from build123d import *

# Parameters (mm, degrees)
BOSS_EXTRUDE1_DEPTH = 4
SKETCH2_R           = 1.95
CUT_EXTRUDE1_DEPTH  = 3
FILLET1_R           = 0.25


with BuildPart() as part:
    # Sketch1 → Boss-Extrude1 (new body)
    with BuildSketch(Plane(origin=(0, 0, 0), x_dir=(1, 0, 0), z_dir=(0, 1, 0))):
        Polygon((2.362917062, -1.848410928), (2.782229351, 1.122140739), (0.419312289, 2.970551667), (-2.362917062, 1.848410928), (-2.782229351, -1.122140739), (-0.419312289, -2.970551667), align=None)
    extrude(amount=BOSS_EXTRUDE1_DEPTH)

    # Sketch2 → Cut-Extrude1 (cut)
    with BuildSketch(Plane(origin=(0, 4, 0), x_dir=(1, 0, 0), z_dir=(0, 1, 0))):
        Circle(SKETCH2_R)
    extrude(amount=-CUT_EXTRUDE1_DEPTH, mode=Mode.SUBTRACT)

    # Fillet1
    fillet1_edges = [part.edges().sort_by_distance(p)[0] for p in [
        (-1.95, 4, 0),
    ]]
    fillet(fillet1_edges, radius=FILLET1_R)


solid = part.part
Source: CAD feature listing. Evaluate the final solid. Frame: model axes, mm. A direction names the side the tool comes from. Give positions to 0.01 mm unless a question says otherwise; leave off trailing zeros. Order: outer loops, then holes, each group sorted by start corner. A loop starts at its lowest first (then second) coordinate and runs counter-clockwise, first axis right, second up. Notation, with made-up numbers: (-29, -16.5) -> (-6, -16.5) arc R29 cw to (-6, 16.5) -> close; hole circle Ø8 at (22.5, 38.5). An arc over 180 degrees is marked (long way). Write item = value, one per line.
Item 1: Set-up query: faces 4 (the face through (-1.62, 1.97, 2.03)), 5 (the face through (-1.437, 2.394, -1.318)). Return all of +Z, -Z, +X, -X, +Y, -Y with unobstructed straight access to the full face (end or side cutting, diameter ignored); none if empty.
Check result:
face_4 = +Z, -X, +Y, -Y
face_5 = +Y
Item 2: Section query C-C (z = 0). Output: boundary loops of the cut face in (x, y), then the cut area to 3 significant figures.
Check result:
outline = (-2.62, 0) -> (2.62, 0) -> (2.62, 4) -> (2.2, 4) arc R0.25 ccw to (1.95, 3.75) -> (1.95, 1) -> (-1.95, 1) -> (-1.95, 3.75) arc R0.25 ccw to (-2.2, 4) -> (-2.62, 4) -> close
area = 9.26 mm²
Item 3: Section query D-D (x = 0). Output: boundary loops of the cut face in (y, z).
Check result:
outline = (0, -2.8) -> (4, -2.8) -> (4, -2.2) arc R0.25 ccw to (3.75, -1.95) -> (1, -1.95) -> (1, 1.95) -> (3.75, 1.95) arc R0.25 ccw to (4, 2.2) -> (4, 2.8) -> (0, 2.8) -> close
Item 4: Section query B-B (y = 0.45). Output: boundary loops of the cut face in (x, z), then the cut area to 3 significant figures.
Check result:
outline = (-2.78, 1.12) -> (-2.36, -1.85) -> (0.42, -2.97) -> (2.78, -1.12) -> (2.36, 1.85) -> (-0.42, 2.97) -> close
area = 23.4 mm²
Item 5: Mould query, pull axis X, two halves, no side actions, for faces 1 (the face through (-1, 2, -2.4)), 2 (the face through (1, 2, 2.4)), 3 (the face through (0, 1, 0)). Classes: +X half, -X half, draft (parallel to the pull), parting line (faces both ways), or undercut.
Check result:
face_1 = -X half
face_2 = +X half
face_3 = undercut
Item 6: Ray query, probe 1 along Y at (x, z) = (-1.1, 1.3); probe 2 along X at (y, z) = (1.85, -1.5); probe 3 along Z at (x, y) = (1.45, 2.1). Return the intervals inside material, ascending.
Check result:
probe_1 = 0 to 1
probe_2 = -2.41 to -1.25, 1.25 to 2.3
probe_3 = -2.16 to -1.3, 1.3 to 2.22
Item 7: Contact query for flat-ended pins moving along their axis: pin 1 (2.5 mm diameter, centred on x = 0, z = 0, fed in from +Y); pin 2 (2 mm diameter, centred on y = 2, z = 1.5, fed in from +X). Output: stop coordinate, or through.
Check result:
pin_1 = 1
pin_2 = 2.55
Item 8: Section query A-A (y = 1.7). Output: boundary loops of the cut face in (x, z).
Check result:
outline = (-2.78, 1.12) -> (-2.36, -1.85) -> (0.42, -2.97) -> (2.78, -1.12) -> (2.36, 1.85) -> (-0.42, 2.97) -> close; hole circle Ø3.9 at (0, 0)
